Check sheet for the modelled part. Datum: model origin and axes. Units: mm. A direction names the side the tool comes from. Coordinates: 2 decimals unless noted, no trailing zeros. Loops run counter-clockwise (first coordinate to the right, second up) from the corner with the lowest first, then second, coordinate; pieces in that order, holes last.
```python
from build123d import *

# Parameters (mm, degrees)
SKETCH1_W           = 200
SKETCH1_H           = 200
BOSS_EXTRUDE1_DEPTH = 10
SKETCH2_W           = 100
SKETCH2_H           = 100
SKETCH2_R           = 40
BOSS_EXTRUDE2_DEPTH = 220
SKETCH3_R           = 50
SKETCH3_R_2         = 40
BOSS_EXTRUDE3_DEPTH = 100


with BuildPart() as part:
    # Sketch1 → Boss-Extrude1 (new body)
    with BuildSketch(Plane(origin=(0, 0, 0), x_dir=(1, 0, 0), z_dir=(0, 1, 0))):
        with Locations((100, 100)):
            Rectangle(SKETCH1_W, SKETCH1_H)
    extrude(amount=BOSS_EXTRUDE1_DEPTH)

    # Sketch2 → Boss-Extrude2 (add)
    with BuildSketch(Plane(origin=(0, 10, 0), x_dir=(1, 0, 0), z_dir=(0, 1, 0))):
        with Locations((100, 100)):
            Rectangle(SKETCH2_W, SKETCH2_H)
        with Locations(Location((100, 100, 0), (0, 0, 270))):
            Circle(SKETCH2_R, mode=Mode.SUBTRACT)
    extrude(amount=BOSS_EXTRUDE2_DEPTH)

    # Sketch3 → Boss-Extrude3 (add)
    with BuildSketch(Plane(origin=(0, 230, 0), x_dir=(1, 0, 0), z_dir=(0, 1, 0))):
        with Locations(Location((100, 100, 0), (0, 0, 270))):
            Circle(SKETCH3_R)
        with Locations(Location((100, 100, 0), (0, 0, 270))):
            Circle(SKETCH3_R_2, mode=Mode.SUBTRACT)
    extrude(amount=BOSS_EXTRUDE3_DEPTH)


solid = part.part
```
1) Scan lines: line 1 (X direction, y = 130.5, z = -100); line 2 (Y direction, x = 171.5, z = -58); line 3 (Z direction, x = 134, y = 83.5). Record each from-to range of solid material in increasing order.
Answer sheet:
line 1: x = 50 to 60, 140 to 150
line 2: y = 0 to 10
line 3: z = -150 to -121.07, -78.93 to -50
2) Depth check by flat-ended pin: pin 1 (10 mm diameter, centred on y = 296.5, z = -73, fed in from +X); pin 2 (25 mm diameter, centred on x = 115, z = -84, fed in from +Y); pin 3 (4 mm diameter, centred on y = 118.5, z = -85, fed in from -X). Enter the tip coordinate at first touch or a pass-through.
Answer sheet:
pin 1: stops at x = 144.9
pin 2: stops at y = 10
pin 3: stops at x = 50
3) Section check C-C on x = 127. Enter the section's corners in (y, z).
Answer sheet:
outline: (0, -200) - (10, -200) - (10, -150) - (230, -150) - (230, -142.08) - (330, -142.08) - (330, -129.51) - (10, -129.51) - (10, -70.49) - (330, -70.49) - (330, -57.92) - (230, -57.92) - (230, -50) - (10, -50) - (10, 0) - (0, 0) - close
4) Section check D-D on y = 286. Enter the section's corners in (x, z), plus the area to 3 significant figures.
Answer sheet:
outline: circle Ø100 at (100, -100); hole circle Ø80 at (100, -100)
area: 2,830 mm2
5) Section check B-B on z = -56. Enter the section's corners in (x, y).
Answer sheet:
outline: (0, 0) - (200, 0) - (200, 10) - (150, 10) - (150, 230) - (123.75, 230) - (123.75, 330) - (76.25, 330) - (76.25, 230) - (50, 230) - (50, 10) - (0, 10) - close
6) Set-up check for faces 1 (the flat face through (140, 230, -60)), 2 (the flat face through (99, 118, -50)), 3 (the flat face through (60, 230, -62)), 4 (the flat face through (99, 118, -150)): record each of +Z, -Z, +X, -X, +Y, -Y from which the full face is reachable in a straight line by a thin tool's end or side.
Answer sheet:
face 1: +Z, +X, +Y
face 2: +Z, +X, -X, +Y
face 3: +Z, -X, +Y
face 4: -Z, +X, -X, +Y
7) Section check A-A on y = 113. Enter the section's corners in (x, z).
Answer sheet:
outline: (50, -150) - (150, -150) - (150, -50) - (50, -50) - close; hole circle Ø80 at (100, -100)
8) Mould release check, pull along Z, two halves, no side actions. Record for faces 5 (the cylindrical face through (112.015, 167.76, -61.847)), 6 (the flat face through (99, 5, 0)), 7 (the flat face through (60, 230, -138)): +Z half, -Z half, draft (parallel to the pull), parting line (faces both ways), or undercut.
Answer sheet:
face 5: undercut
face 6: +Z half
face 7: draft
